Could you check a few things on this model? Use its own coordinates, in mm. Coordinates: 2 decimals unless noted, no trailing zeros. Order: outer loops, then holes, each group sorted by start corner. A loop starts at its lowest first (then second) coordinate and runs counter-clockwise, first axis right, second up.
```python
from build123d import *

# Parameters (mm, degrees)
BOX_W             = 241
BOX_H             = 20
BOX_DEPTH         = 3
CYLINDER_R        = 2.25
CYLINDER_DEPTH    = 3
CYLINDER001_R     = 2.25
CYLINDER001_DEPTH = 3
CYLINDER002_R     = 2.25
CYLINDER002_DEPTH = 3
CYLINDER003_R     = 2.25
CYLINDER003_DEPTH = 3


with BuildPart() as part:
    # Box → Box (join)
    with BuildSketch(Plane.XY):
        with Locations((120.5, 10)):
            Rectangle(BOX_W, BOX_H)
    extrude(amount=BOX_DEPTH)

    # Cylinder → Cylinder (cut)
    with BuildSketch(Plane(origin=(7, 10, 0), x_dir=(1, 0, 0), z_dir=(0, 0, 1))):
        Circle(CYLINDER_R)
    extrude(amount=CYLINDER_DEPTH, mode=Mode.SUBTRACT)

    # Cylinder001 → Cylinder001 (cut)
    with BuildSketch(Plane(origin=(234, 10, 0), x_dir=(1, 0, 0), z_dir=(0, 0, 1))):
        Circle(CYLINDER001_R)
    extrude(amount=CYLINDER001_DEPTH, mode=Mode.SUBTRACT)

    # Cylinder002 → Cylinder002 (cut)
    with BuildSketch(Plane(origin=(89, 10, 0), x_dir=(1, 0, 0), z_dir=(0, 0, 1))):
        Circle(CYLINDER002_R)
    extrude(amount=CYLINDER002_DEPTH, mode=Mode.SUBTRACT)

    # Cylinder003 → Cylinder003 (cut)
    with BuildSketch(Plane(origin=(155, 10, 0), x_dir=(1, 0, 0), z_dir=(0, 0, 1))):
        Circle(CYLINDER003_R)
    extrude(amount=CYLINDER003_DEPTH, mode=Mode.SUBTRACT)


solid = part.part
```
Item 1: Thinking about a two-plate mould opening in X: for faces 1 (the face through (233.71, 12.23, 1.48)), 2 (the face through (119, 10, 3)), which applies, +X half, -X half, draft (parallel to the pull), parting line (faces both ways), or undercut?
Item 2: Suppose I cut it at B-B (x = 234). List the corners of the cut face in (y, z) for me, and give its area (3 significant figures).
Item 3: Suppose I cut it at A-A (y = 10). List the corners of the cut face in (x, z) for me.
Item 4: I need wall thicknesses on line 1 (X direction, y = 11.75, z = 1.3); line 2 (Y direction, x = 234, z = 2.45); line 3 (X direction, y = 9, z = 1.7). Which ranges of each line are inside material? Lowest first, please.
Item 5: For pin 1 Ø5 at (x, y) = (89, 10) entering from -Z; pin 2 Ø2.5 at (x, y) = (234, 10) entering from +Z, each with a flat end and sliding along its axis, tell me the tip position at first contact or that it passes through.
Geometry results:
1. face 1: undercut
1. face 2: draft
2. outline: (0, 0) - (7.75, 0) - (7.75, 3) - (0, 3) - close; (12.25, 0) - (20, 0) - (20, 3) - (12.25, 3) - close
2. area: 46.5 mm2
3. outline: (0, 0) - (4.75, 0) - (4.75, 3) - (0, 3) - close; (9.25, 0) - (86.75, 0) - (86.75, 3) - (9.25, 3) - close; (91.25, 0) - (152.75, 0) - (152.75, 3) - (91.25, 3) - close; (157.25, 0) - (231.75, 0) - (231.75, 3) - (157.25, 3) - close; (236.25, 0) - (241, 0) - (241, 3) - (236.25, 3) - close
4. line 1: x = 0 to 5.59, 8.41 to 87.59, 90.41 to 153.59, 156.41 to 232.59, 235.41 to 241
4. line 2: y = 0 to 7.75, 12.25 to 20
4. line 3: x = 0 to 4.98, 9.02 to 86.98, 91.02 to 152.98, 157.02 to 231.98, 236.02 to 241
5. pin 1: stops at z = 0
5. pin 2: passes through
